from build123d import *

# Parameters (mm, degrees)
F0_R     = 85
F1_DEPTH = 10
F3_DEPTH = 10
F4_R     = 5
F4_R_2   = 1.5
F5_DEPTH = 10.001


# Not quite as in the source:
# - a feature names something its author has since deleted; it is built from what else it names


with BuildPart() as f1:
    # F0 (on Front) → F1 (new body)
    with BuildSketch(Plane.XZ):
        Circle(F0_R)
    extrude(amount=F1_DEPTH)

    # F2 (on face) → F3 (join)
    with BuildSketch(Plane.XZ.offset(10)):
        with BuildLine():
            Line((0, 88), (0, 85))
            ThreePointArc((0, 85), (10.0709372009, 84.4012809375), (20, 82.6135582093))
            ThreePointArc((20, 82.6135582093), (14.3075201815, 93.5944770544), (2.75, 98))
            Line((2.75, 98), (2.75, 88))
            Line((2.75, 88), (0, 88))
        make_face()
        with BuildLine():
            ThreePointArc((-85, 0), (-84.4012809375, 10.0709372009), (-82.6135582093, 20))
            ThreePointArc((-82.6135582093, 20), (-93.5944770544, 14.3075201815), (-98, 2.75))
            Line((-98, 2.75), (-88, 2.75))
            Line((-88, 2.75), (-88, 0))
            Line((-88, 0), (-85, 0))
        make_face()
        with BuildLine():
            ThreePointArc((0, -85), (-10.0709372009, -84.4012809375), (-20, -82.6135582093))
            ThreePointArc((-20, -82.6135582093), (-14.3075201815, -93.5944770544), (-2.75, -98))
            Line((-2.75, -98), (-2.75, -88))
            Line((-2.75, -88), (0, -88))
            Line((0, -88), (0, -85))
        make_face()
        with BuildLine():
            Line((88, 0), (85, 0))
            ThreePointArc((85, 0), (84.4012809375, -10.0709372009), (82.6135582093, -20))
            ThreePointArc((82.6135582093, -20), (93.5944770544, -14.3075201815), (98, -2.75))
            Line((98, -2.75), (88, -2.75))
            Line((88, -2.75), (88, 0))
        make_face()
    extrude(amount=-F3_DEPTH)

    # F4 (on face) → F5 (cut, through all)
    with BuildSketch(Plane.XZ.offset(10)):
        Circle(F4_R)
        with Locations((0, 30)):
            Circle(F4_R_2)
        with Locations((30, 0)):
            Circle(F4_R_2)
        with Locations((-30, 0)):
            Circle(F4_R_2)
        with Locations((0, -30)):
            Circle(F4_R_2)
    extrude(amount=-F5_DEPTH, mode=Mode.SUBTRACT)


solid = f1.part
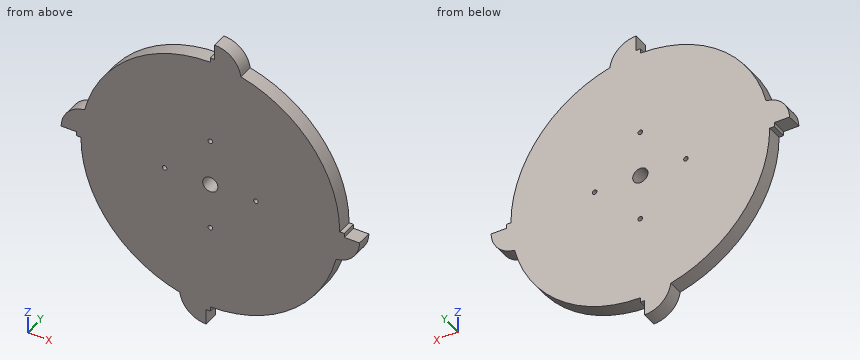
Can you work these out from the model? Positions are in its coordinate system, mm. Round coordinates to 2 decimals unless told otherwise and drop trailing zeros. Loops run counter-clockwise (first coordinate to the right, second up) from the corner with the lowest first, then second, coordinate; pieces in that order, holes last. Notation, with made-up numbers: (5.5, 64.25) - (27.5, 64.25) arc R13 ccw to (27.5, 81.25) - close; hole circle Ø7 at (-36.75, 17). An arc over 180 degrees is marked (long way). Use CSV: the item, a comma, the result in double quotes. Start each with the question number.
1) For pin 1 Ø1.5 at (y, z) = (-5, -87) entering from +X; pin 2 Ø1.5 at (y, z) = (-5.5, -59) entering from -X; pin 3 Ø2.5 at (x, z) = (30, 0) entering from +Y; pin 4 Ø4 at (x, y) = (52.5, -3) entering from +Z, each with a flat end and sliding along its axis, tell me the tip position at first contact or that it passes through.
2) If we section it at A-A on y = -4: Write out the boundary of the cut face in (x, z), plus the area to 3 significant figures.
3) If we section it at C-C on z = -43: Write out the boundary of the cut face in (x, y), plus the area to 3 significant figures.
4) Please list where these lines run through material, in increasing order: probe 1 along X at (y, z) = (-5.75, -1); probe 2 along Z at (x, y) = (-30, -5.75); probe 3 along Z at (x, y) = (55.5, -2). Write a range as [from, to].
5) If we section it at B-B on x = 45: Write out the boundary of the cut face in (y, z).
Geometry results:
1,pin 1,"stops at x = 0"
1,pin 2,"stops at x = -61.9"
1,pin 3,"passes through"
1,pin 4,"stops at z = 68.37"
2,outline,"(-98, 2.75) - (-88, 2.75) - (-88, 0) - (-85, 0) arc R85 ccw to (-20, -82.61) arc R17.36 ccw to (-2.75, -98) - (-2.75, -88) - (0, -88) - (0, -85) arc R85 ccw to (82.61, -20) arc R17.36 ccw to (98, -2.75) - (88, -2.75) - (88, 0) - (85, 0) arc R85 ccw to (20, 82.61) arc R17.36 ccw to (2.75, 98) - (2.75, 88) - (0, 88) - (0, 85) arc R85 ccw to (-82.61, 20) arc R17.36 ccw to start; hole circle Ø3 at (-30, 0); hole circle Ø10 at (0, 0); hole circle Ø3 at (0, -30); hole circle Ø3 at (0, 30); hole circle Ø3 at (30, 0)"
2,area,"23,300 mm2"
3,outline,"(-73.32, -10) - (73.32, -10) - (73.32, 0) - (-73.32, 0) - close"
3,area,"1,470 mm2"
4,probe 1,"x = [-84.99, -31.12], [-28.88, -4.9], [4.9, 28.88], [31.12, 88]"
4,probe 2,"z = [-79.53, -1.5], [1.5, 79.53]"
4,probe 3,"z = [-64.38, 64.38]"
5,outline,"(-10, -72.11) - (0, -72.11) - (0, 72.11) - (-10, 72.11) - close"
